Can you work these out from the model? Positions are in its coordinate system, mm. A direction names the side the tool comes from. Coordinates: 2 decimals unless noted, no trailing zeros. Order: outer loops, then holes, each group sorted by start corner. A loop starts at its lowest first (then second) coordinate and runs counter-clockwise, first axis right, second up. Notation, with made-up numbers: (13.5, -7) - (49.5, -7) arc R20 ccw to (49.5, -1) - close; hole circle Ø1 at (-8.75, -28). An arc over 180 degrees is marked (long way). Use a Markdown table: item, result. Add a question column.
(1) I want a section at A-A (z = -2.5). List the corners of the cut face in (x, y) for me (3 decimals).
(2) If I drill on L1, parallel to X at y = 0.25, z = -1.5; L2, parallel to Z at x = 11.5, y = -1.5, over which ranges is the centre line in solid material (lowest first)? Write a range as [from, to].
(3) We'd pull the mould along X, two halves only. Please class faces 3 (the flat face through (-14, 0, 0)), 4 (the flat face through (17, 0, 0)), 5 (the flat face through (0, 0, -17)): pulls with the +X half, pulls with the -X half, needs draft (parallel to the pull), parting line crosses it, or undercut.
(4) I want a section at D-D (x = 15.5). List the corners of the cut face in (y, z) for me (3 decimals), and give its area (3 significant figures).
(5) I want a section at B-B (x = 3). List the corners of the cut face in (y, z) for me (3 decimals), and give its area (3 significant figures).
(6) I want a section at C-C (y = 2.5). List the corners of the cut face in (x, z) for me.
(7) On a 3-axis mill with a long thin cutter (end or side, diameter ignored), from which of +Z, -Z, +X, -X, +Y, -Y can I reach the whole of each face in a straight line? I mean faces 1 (the cylindrical face through (-14.15, -0.05, -13.99)), 2 (the cylindrical face through (-11.9, -0.1, 12)). Say none if no direction works.
Autodesk Inventor part; units mm, degrees
ref_plane "YZ Plane" through (0, 0, 0) normal (1, 0, 0) x (0, 1, 0)
ref_plane "XZ Plane" through (0, 0, 0) normal (0, 1, 0) x (-1, 0, 0)
ref_plane "XY Plane" through (0, 0, 0) normal (0, 0, 1) x (1, 0, 0)
sketch "Sketch1" plane through (0, 0, 0) normal (0, 1, 0) x (-1, 0, 0)
  line L0 (-7, 17) -> (7, 17)
  line L1 (17, 7) -> (17, -7)
  line L2 (7, -17) -> (-7, -17)
  line L3 (-17, -7) -> (-17, 7)
  line L4 (-17, 17) -> (17, -17) construction
  line L5 (17, 17) -> (-17, -17) construction
  arc A0 (7, -17) -> (17, -7) centre (7, -7) ccw
  arc A1 (-17, -7) -> (-7, -17) centre (-7, -7) ccw
  arc A2 (-7, 17) -> (-17, 7) centre (-7, 7) ccw
  arc A3 (17, 7) -> (7, 17) centre (7, 7) ccw
  line L6 (14, -7) -> (14, 7)
  arc A4 (14, 7) -> (7, 14) centre (7, 7) ccw
  line L7 (7, 14) -> (-7, 14)
  arc A5 (-7, 14) -> (-14, 7) centre (-7, 7) ccw
  line L8 (-14, 7) -> (-14, -7)
  arc A6 (-14, -7) -> (-7, -14) centre (-7, -7) ccw
  line L9 (-7, -14) -> (7, -14)
  arc A7 (7, -14) -> (14, -7) centre (7, -7) ccw
  point P0 (0, 0)
  dimension "d0" = 34
  dimension "d1" = 10
  dimension "d2" = 3
extrude "Extrusion1" add sketch "Sketch1" along normal mid plane 7.75
properties part number "tenzo"
Answers follow:
| question | item | result |
|---|---|---|
| 1 | outline | (-17, -3.875) - (-14, -3.875) - (-14, 3.875) - (-17, 3.875) - close; (14, -3.875) - (17, -3.875) - (17, 3.875) - (14, 3.875) - close |
| 2 | L1 | x = [-17, -14], [14, 17] |
| 2 | L2 | z = [-15.93, -12.36], [12.36, 15.93] |
| 3 | face 3 | undercut |
| 3 | face 4 | pulls with the +X half |
| 3 | face 5 | needs draft |
| 4 | outline | (-3.875, -12.268) - (3.875, -12.268) - (3.875, 12.268) - (-3.875, 12.268) - close |
| 4 | area | 190 mm² |
| 5 | outline | (-3.875, -17) - (3.875, -17) - (3.875, -14) - (-3.875, -14) - close; (-3.875, 14) - (3.875, 14) - (3.875, 17) - (-3.875, 17) - close |
| 5 | area | 46.5 mm² |
| 6 | outline | (-17, -7) arc R10 ccw to (-7, -17) - (7, -17) arc R10 ccw to (17, -7) - (17, 7) arc R10 ccw to (7, 17) - (-7, 17) arc R10 ccw to (-17, 7) - close; hole (-14, -7) arc R7 ccw to (-7, -14) - (7, -14) arc R7 ccw to (14, -7) - (14, 7) arc R7 ccw to (7, 14) - (-7, 14) arc R7 ccw to (-14, 7) - close |
| 7 | face 1 | -Z, -X, +Y, -Y |
| 7 | face 2 | +Y, -Y |
